```python
from build123d import *

# Parameters (mm, degrees)
BOSS_EXTRU_1_DEPTH      = 6
BOSS_EXTRU_1_DEPTH_BACK = 4
ESQUISSE1_R             = 5
BOSS_EXTRU_2_DEPTH      = 5
BOSS_EXTRU_2_DEPTH_BACK = 1
ESQUISSE2_R             = 3
ESQUISSE3_R             = 1.5
ENL_V_MAT_EXTRU_2_DEPTH = 10
ESQUISSE4_R             = 2.5
ENL_V_MAT_EXTRU_3_DEPTH = 5
CONG_1_R                = 0.8


with BuildPart() as part:
    # Esquisse1 → Boss.-Extru.1 (new, two sides: drawn at the far end of the back side and taken through both)
    with BuildSketch(Plane(origin=(0, 0, 0), x_dir=(1, 0, 0), z_dir=(0, 1, 0)).offset(-BOSS_EXTRU_1_DEPTH_BACK)):
        with Locations(Location((0, 0, 0), (0, 0, 270))):
            Circle(ESQUISSE1_R)
    extrude(amount=BOSS_EXTRU_1_DEPTH + BOSS_EXTRU_1_DEPTH_BACK)

    # Esquisse2 → Boss.-Extru.2 (add, two sides: drawn at the far end of the back side and taken through both)
    with BuildSketch(Plane(origin=(0, 6, 0), x_dir=(1, 0, 0), z_dir=(0, 1, 0)).offset(-BOSS_EXTRU_2_DEPTH_BACK)):
        with Locations(Location((0, 0, 0), (0, 0, 270))):
            Circle(ESQUISSE2_R)
    extrude(amount=BOSS_EXTRU_2_DEPTH + BOSS_EXTRU_2_DEPTH_BACK)

    # Esquisse3 → Enlèv. mat.-Extru.2 (cut)
    with BuildSketch(Plane(origin=(0, 11, 0), x_dir=(1, 0, 0), z_dir=(0, 1, 0))):
        with Locations(Location((0, 0, 0), (0, 0, 270))):
            Circle(ESQUISSE3_R)
    extrude(amount=-ENL_V_MAT_EXTRU_2_DEPTH, mode=Mode.SUBTRACT)

    # Esquisse4 → Enlèv. mat.-Extru.3 (cut)
    with BuildSketch(Plane.XZ.offset(4)):
        with Locations(Location((0, 0, 0), (0, 0, 270))):
            Circle(ESQUISSE4_R)
    extrude(amount=-ENL_V_MAT_EXTRU_3_DEPTH, mode=Mode.SUBTRACT)

    # Congé1
    cong_1_edges = [part.edges().sort_by_distance(p)[0] for p in [
        (0, 11, -1.5),
    ]]
    fillet(cong_1_edges, radius=CONG_1_R)


solid = part.part
```
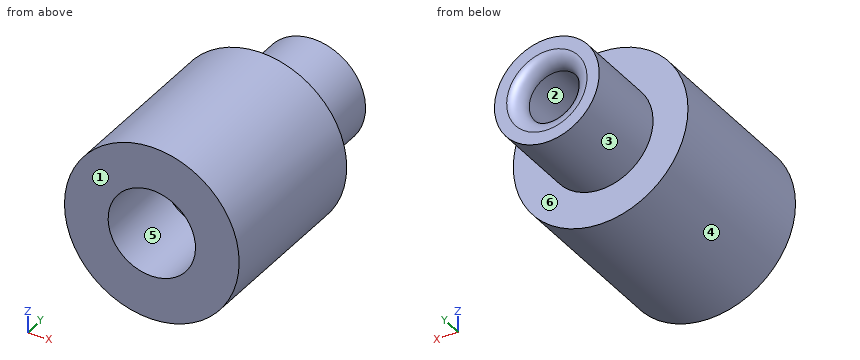
Design review of the part built by this model. Coordinates are the model's own, in mm. Face numbers are marked on the shaded views. A direction names the side the tool comes from. Give positions to 0.01 mm unless a question says otherwise; leave off trailing zeros. Loops run counter-clockwise (first coordinate to the right, second up) from the corner with the lowest first, then second, coordinate; pieces in that order, holes last. Notation, with made-up numbers: (74.5, 81.5) -> (109.5, 81.5) arc R12 ccw to (109.5, 100.5) -> close; hole circle Ø1 at (-33.75, 1). An arc over 180 degrees is marked (long way). Write each question's results on one line, items separated by ' | '.
Q1. Machinability: for the marked faces 4, 5 and 6, which of the approach directions +Z, -Z, +X, -X, +Y, -Y give a long, thin tool a straight path to every point of the face, cutting with its end or side? Answer none if there is none.
Reply:
face 4: +Y, -Y | face 5: -Y | face 6: +Y
Q2. For pin 1 Ø5 at (y, z) = (2.5, -4) entering from -X; pin 2 Ø6 at (x, y) = (3.5, 8) entering from +Z; pin 3 Ø2 at (y, z) = (-2, -2) entering from -X; pin 4 Ø1.8 at (x, z) = (0, 0) entering from +Y, all flat-tipped, find the tip position at first contact; note any pin that passes through.
Reply:
pin 1: stops at x = -4.77 | pin 2: stops at z = 4.84 | pin 3: stops at x = -4.9 | pin 4: passes through
Q3. Take a section at C-C, the plane y = -1.5. Write out the cut boundary in (x, z).
Reply:
outline: circle Ø10 at (0, 0); hole circle Ø5 at (0, 0)
Q4. Take a section at D-D, the plane x = -4. Write out the cut boundary in (y, z).
Reply:
outline: (-4, -3) -> (6, -3) -> (6, 3) -> (-4, 3) -> close
Q5. The part is to be moulded in two halves that separate along X. For the marked faces 1, 2 and 3, say which applies: +X half, -X half, draft (parallel to the pull), parting line (faces both ways), or undercut.
Reply:
face 1: draft | face 2: undercut | face 3: parting line
Q6. Take a section at A-A, the plane z = 0. Write out the cut boundary in (x, y), plus the area to 3 significant figures.
Reply:
outline: (-5, -4) -> (-2.5, -4) -> (-2.5, 1) -> (-1.5, 1) -> (-1.5, 10.2) arc R0.8 ccw to (-2.3, 11) -> (-3, 11) -> (-3, 6) -> (-5, 6) -> close; (1.5, 1) -> (2.5, 1) -> (2.5, -4) -> (5, -4) -> (5, 6) -> (3, 6) -> (3, 11) -> (2.3, 11) arc R0.8 ccw to (1.5, 10.2) -> close | area: 74.7 mm²
Q7. Wall thickness on L1, parallel to X at y = 5.5, z = 0; L2, parallel to X at y = 8.5, z = 0; L3, parallel to Y at x = 3.75, z = 2.75: over which ranges is each line inside the solid? List them lowest first.
Reply:
L1: x = -5 to -1.5, 1.5 to 5 | L2: x = -3 to -1.5, 1.5 to 3 | L3: y = -4 to 6
Q8. Take a section at B-B, the plane x = 0. Write out the cut boundary in (y, z), plus the area to 3 significant figures.
Reply:
outline: (-4, -5) -> (6, -5) -> (6, -3) -> (11, -3) -> (11, -2.3) arc R0.8 ccw to (10.2, -1.5) -> (1, -1.5) -> (1, -2.5) -> (-4, -2.5) -> close; (-4, 2.5) -> (1, 2.5) -> (1, 1.5) -> (10.2, 1.5) arc R0.8 ccw to (11, 2.3) -> (11, 3) -> (6, 3) -> (6, 5) -> (-4, 5) -> close | area: 74.7 mm²
